Answer from the drawing. Dimensions are ordinates in mm from the lowest x, y and z of the part. A direction names the side the tool comes from. Coordinates: 2 decimals unless noted, no trailing zeros. Loops run counter-clockwise (first coordinate to the right, second up) from the corner with the lowest first, then second, coordinate; pieces in that order, holes last.
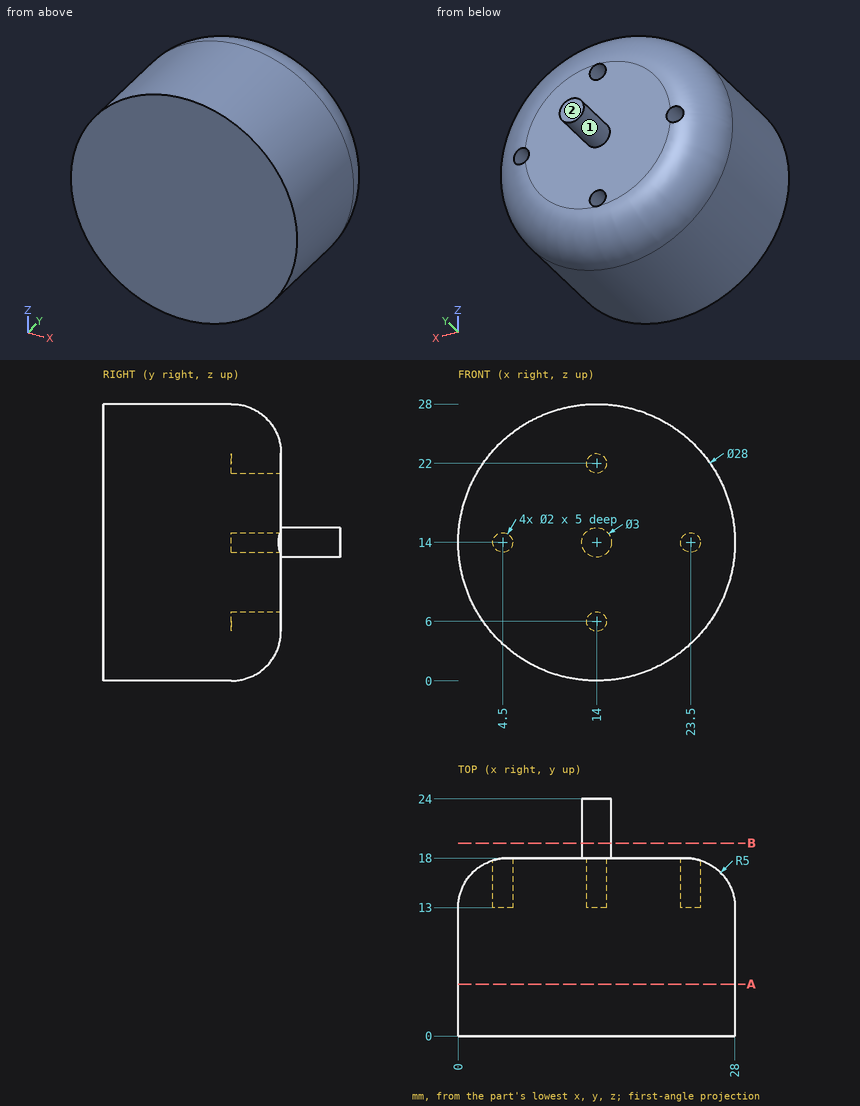
Item 1: Which of the six approach directions +Z, -Z, +X, -X, +Y, -Y give full straight-line access (tool end or side, diameter ignored) to the marked faces 1 and 2?
Numbers:
face 1: +Y
face 2: +Z, -Z, +X, -X, +Y
Item 2: Find the intervals of material crossed by line 1 along Z through (x, y) = (14, 15.05); line 2 along Y through (x, z) = (16.75, 19.5); line 3 along Z through (x, y) = (4.5, 14.25), in increasing order.
Numbers:
line 1: z = 0.44 to 5, 7 to 21, 23 to 27.56
line 2: y = 0 to 18
line 3: z = 3.93 to 13, 15 to 24.07
Item 3: Given pin 1 (4 mm diameter, centred on x = 9.5, z = 5.5, fed in from +Y); pin 2 (5 mm diameter, centred on y = 11, z = 21, fed in from +X); pin 3 (0.6 mm diameter, centred on x = 14, z = 6, fed in from +Y), each flat-ended and moving along its own axis, determine where each tip first touches the part or whether it passes through.
Numbers:
pin 1: stops at y = 18
pin 2: stops at x = 27.26
pin 3: stops at y = 13
Item 4: A cutting plane is placed at A-A on y = 5.25. Determine the outline of the cut face in (x, z).
Numbers:
outline: circle Ø28 at (14, 14)
Item 5: A cutting plane is placed at B-B on y = 19.5. Determine the outline of the cut face in (x, z), then the cut area to 3 significant figures.
Numbers:
outline: circle Ø3 at (14, 14)
area: 7.07 mm2
